The listing builds one solid part. Answer for the finished solid, in the listing's coordinates (mm). A direction names the side the tool comes from. Coordinates: 2 decimals unless noted, no trailing zeros.
(1) Which of the six approach directions +Z, -Z, +X, -X, +Y, -Y give full straight-line access (tool end or side, diameter ignored) to faces 5 (the flat face through (2, -9, 0)), 6 (the flat face through (31.1, -43.4, -1.5)), 7 (the cylindrical face through (2.405, -17.973, -1.521)), 8 (the flat face through (-2, -6, -0.5))?
(2) Straight lines are drawn through the part: line 1 (X direction, y = -34, z = -3.5); line 2 (X direction, y = -4.25, z = 1.4); line 3 (Z direction, x = 11, y = -18). For each, find the intervals that lie inside material, in ascending order.
(3) Given P1, Ø1, axis at x = 13, y = -19, coming from the -Z side; P2, Ø1.5, axis at y = -49, z = -6, coming from the +X side (3 decimals); P3, Ø2, axis at x = 1.5, y = -4.5, coming from the -Z side, each flat-ended and moving along its own axis, determine where each tip first touches the part or whether it passes through.
(4) For a pull along Y with two mould halves and no side action, classify faces 1 (the flat face through (25.423, -22.066, 0.042)), 2 (the cylindrical face through (-4.155, 0.748, 1.479)), 3 (the cylindrical face through (34.8, -48.2, -4)), 4 (the flat face through (35, -48, -10)) as +Y half, -Y half, draft (parallel to the pull), parting line (faces both ways), or undercut.
Autodesk Inventor part; units mm, degrees
ref_plane "YZ Plane" through (0, 0, 0) normal (1, 0, 0) x (0, 1, 0)
ref_plane "XY Plane" through (0, 0, 0) normal (0, 0, 1) x (1, 0, 0)
sketch "Skizze1" plane through (0, 0, 0) normal (0, 0, 1) x (1, 0, 0)
  line L0 (23.3115, -64.9198) -> (53.8426, -40.6536)
  circle A0 centre (0, -4.25) radius 6.5
  line L1 (43.6656, -48.7423) -> (33.4885, -56.8311)
  line L2 (33.4885, -56.8311) -> (-5.0885, -8.2944)
  line L3 (-5.0885, -8.2944) -> (5.0885, -0.2056)
  line L4 (5.0885, -0.2056) -> (43.6656, -48.7423)
  point P0 (0, 0)
  dimension "d0" = 13
extrude "Extrusion1" add sketch "Skizze1" along normal blind 3
sketch "Skizze2" plane through (43.6656, -48.7423, 0) normal (0.6222102, -0.7828502, 0) x (0.7828502, 0.6222102, 0)
  circle A0 centre (-17.7583, -20) radius 1.5
  circle A1 centre (4.7583, -20) radius 1.5
  circle A2 centre (-6.5, -0.5) radius 1.5
  line L0 (-23, -30.5) -> (10, -30.5)
  line L1 (10, -30.5) -> (10, -26.4615)
  arc A3 (11.0169, -22.0678) -> (10, -26.4615) centre (20, -26.4615) ccw
  arc A4 (11.0169, -22.0678) -> (-24.0169, -22.0678) centre (-6.5, -13.5) ccw
  arc A5 (-23, -26.4615) -> (-24.0169, -22.0678) centre (-33, -26.4615) ccw
  line L2 (-23, -26.4615) -> (-23, -30.5)
  line L3 (12.6833, -10) -> (-25.6833, -10)
  line L4 (-104.8912, -12) -> (94.8547, -12)
  line L5 (-13, 3) -> (0, 3)
  line L6 (3.8923, 3) -> (-16.8923, 3)
  line L7 (-21.75, -5.4123) -> (-19, -3.8246)
  line L8 (-19, -3.8246) -> (-16.25, -5.4123)
  line L9 (-16.25, -5.4123) -> (-16.25, -8.5877)
  line L10 (-16.25, -8.5877) -> (-19, -10.1754)
  line L11 (-19, -10.1754) -> (-21.75, -8.5877)
  line L12 (-21.75, -8.5877) -> (-21.75, -5.4123)
  line L13 (3.25, -5.4123) -> (6, -3.8246)
  line L14 (6, -3.8246) -> (8.75, -5.4123)
  line L15 (8.75, -5.4123) -> (8.75, -8.5877)
  line L16 (8.75, -8.5877) -> (6, -10.1754)
  line L17 (6, -10.1754) -> (3.25, -8.5877)
  line L18 (3.25, -8.5877) -> (3.25, -5.4123)
  circle A6 centre (-6.5, -13.5) radius 5
  point P0 (-3.8556, 0)
  dimension "d3" = 2
extrude "Extrusion2" add sketch "Skizze2" against normal blind 12 contours A4 L6 L5 L3 L16 L15 L14 L13 L18 L17 A6 L10 L9 L8 L7 L12 L11 | L11 L12 L7 L8 L9 L10 L3 | A6 L3 | L3 L17 L18 L13 L14 L15 L16
sketch "Skizze3" plane through (0, 0, 3) normal (0, 0, 1) x (1, 0, 0)
  line L0 (36.199, -39.3481) -> (5.0885, -0.2056)
  arc A0 (5.0885, -0.2056) -> (-5.0885, -8.2944) centre (0, -4.25) ccw
  line L1 (-5.0885, -8.2944) -> (26.022, -47.4369)
  line L2 (22.9749, -49.8587) -> (26.022, -47.4369)
  line L3 (30.4414, -59.2529) -> (22.9749, -49.8587)
  line L4 (46.7127, -46.3205) -> (30.4414, -59.2529)
  line L5 (46.7127, -46.3205) -> (39.2461, -36.9263)
  line L6 (36.199, -39.3481) -> (39.2461, -36.9263)
  line L7 (22.9749, -49.8587) -> (-5.0885, -8.2944)
  line L8 (39.2461, -36.9263) -> (5.0885, -0.2056)
  point P0 (0, 0)
extrude "Extrusion3" add sketch "Skizze3" against normal up to surface (3 mm away) contours L0 L8 L6 | L1 L2 L7
sketch "Skizze4" plane through (23.5594, -64.7228, -10) normal (0.6222102, -0.7828502, 0) x (0.7828502, 0.6222102, 0)
  line L0 (29.5756, 13) -> (8.791, 13)
  arc A0 (8.791, 13) -> (0, 0) centre (19.1833, -3.5) ccw
  line L1 (0, 0) -> (38.3667, 0)
  arc A1 (38.3667, 0) -> (29.5756, 13) centre (19.1833, -3.5) ccw
  arc A2 (17.7691, 10) -> (20.5975, 10) centre (19.1833, 9.5) ccw
  line L2 (17.7691, 10) -> (20.5975, 10)
  circle A3 centre (19.1833, 9.5) radius 1.5
  circle A4 centre (19.1833, 9.5) radius 3.5
  point P0 (21.8277, 10)
  dimension "d8" = 7
extrude "Extrusion4" cut sketch "Skizze4" against normal blind 12 contours A4 | L2 A2 | A3 L2
sketch "Skizze6" plane through (23.5594, -64.7228, -10) normal (0.6222102, -0.7828502, 0) x (0.7828502, 0.6222102, 0)
  circle A0 centre (19.1833, 9.5) radius 3.5
  line L0 (29.5756, 13) -> (19.1833, 13) construction
  arc A1 (8.791, 13) -> (0, 0) centre (19.1833, -3.5) ccw construction
  line L1 (0, 0) -> (38.3667, 0) construction
  arc A2 (38.3667, 0) -> (29.5756, 13) centre (19.1833, -3.5) ccw construction
  line L2 (15.6833, 13) -> (22.6833, 13)
  line L3 (22.6833, 13) -> (22.6833, 9.5)
  line L4 (22.6833, 9.5) -> (15.6833, 9.5)
  line L5 (15.6833, 9.5) -> (15.6833, 13)
  circle A3 centre (19.1833, 9.5) radius 3.5
  line L6 (19.1833, 13) -> (8.791, 13)
  point P0 (21.8277, 10)
  point P1 (21.0706, 13)
  point P2 (17.4651, 13)
extrude "Extrusion6" cut sketch "Skizze6" against normal up to surface (12 mm away) contours L4 A0 | A0 L2 L3 | A0 L5 L2 picked at (20.0662, 10.487)
sketch "Skizze7" plane through (36.199, -39.3481, 0) normal (-0.6222102, 0.7828502, 0) x (0.7828502, 0.6222102, 0)
  line L0 (-16.8923, -3) -> (-16.8923, 0)
  line L1 (-16.8923, 0) -> (-10, 0)
  line L2 (3.8923, 0) -> (3.8923, -3)
  arc A0 (3.8923, -3) -> (12.6833, 10) centre (-6.5, 13.5) ccw
  line L3 (12.6833, 10) -> (-25.6833, 10)
  arc A1 (-25.6833, 10) -> (-16.8923, -3) centre (-6.5, 13.5) ccw
  circle A2 centre (-19, 7) radius 1.5
  circle A3 centre (6, 7) radius 1.5
  line L4 (-3, 0.5) -> (-3, 0)
  line L5 (3.8923, 0) -> (-3, 0)
  line L6 (-10, 0) -> (-10, 0.5)
  arc A4 (-3, 0.5) -> (-10, 0.5) centre (-6.5, 0.5) ccw
  point P0 (-3.8556, 0)
extrude "Extrusion7" cut sketch "Skizze7" against normal through all contours A2 | A3
sketch "Skizze8" plane through (0, 0, 0) normal (0, 0, -1) x (-1, 0, 0)
  line L0 (-22.9749, -49.8587) -> (-28.3705, -45.5702)
  line L1 (-22.9749, -49.8587) -> (5.0885, -8.2944)
  arc A0 (5.0885, -8.2944) -> (-5.0885, -0.2056) centre (0, -4.25) ccw
  line L2 (-5.0885, -0.2056) -> (-39.2461, -36.9263)
  circle A1 centre (0, -4.25) radius 3.5
  line L3 (-33.8505, -41.2148) -> (-28.3705, -45.5702)
  line L4 (-39.2461, -36.9263) -> (-33.8505, -41.2148)
  point P0 (0, 0)
  dimension "d17" = 7
extrude "Extrusion8" add sketch "Skizze8" along normal blind 0.5 contours A1
chamfer "Fase1" distance 0.5 angle 45 1 edges at (3.5, -4.25, 0)
sketch "Skizze9" plane through (0, 0, 3) normal (0, 0, 1) x (1, 0, 0)
  circle A0 centre (0, -4.25) radius 3.5
  point P0 (0, 0)
hole "Bohrung1" at (0, -4.25, 3) direction (0, 0, -1) diameter 4 end through all
sketch "Skizze10" plane through (0, 0, 3) normal (0, 0, 1) x (1, 0, 0)
  circle A0 centre (24.2662, -34.7812) radius 3.5
  point P0 (0, 0)
  dimension "d30" = 7
extrude "Extrusion9" cut sketch "Skizze10" against normal through all
sketch "Skizze11" plane through (0, 0, 0) normal (0, 0, -1) x (-1, 0, 0)
  circle A0 centre (-24.2662, -34.7812) radius 3.5
  line L0 (-22.9749, -49.8587) -> (-28.3705, -45.5702)
  line L1 (-22.9749, -49.8587) -> (5.0885, -8.2944)
  arc A1 (5.0885, -8.2944) -> (-5.0885, -0.2056) centre (0, -4.25) ccw
  line L2 (-5.0885, -0.2056) -> (-39.2461, -36.9263)
  circle A2 centre (0, -4.25) radius 4
  arc A3 (-12.4206, -8.0879) -> (-0.9354, -17.2163) centre (0, -4.25) ccw
  line L3 (-22.9749, -49.8587) -> (5.0885, -8.2944)
  line L4 (-33.8505, -41.2148) -> (-28.3705, -45.5702)
  line L5 (-39.2461, -36.9263) -> (-33.8505, -41.2148)
  point P0 (0, 0)
  dimension "d33" = 13
extrude "Extrusion10" add sketch "Skizze11" along normal blind 5 contours L0 L4 L5 L2 A3 L1
fillet "Rundung1" radius 2 2 edges at (0.9354, -17.2163, -2.5) (12.4206, -8.0879, -2.5)
fillet "Rundung2" radius 2 8 edges at (2.4138, -17.9483, -5) (8.0887, -14.4271, -5) (12.8, -9.6934, -5) (26.8705, -23.6221, -5) (12.8073, -34.7996, -5) (22.9749, -49.8587, -1) (39.2461, -36.9263, -1) (31.1105, -43.3925, -5)
fillet "Rundung2" radius 4 2 edges at (49.8614, -36.1536, -10) (19.8261, -60.0257, -10)
properties part number "Mount_B" material "ABS-Kunststoff"
Model answer:
1. face 5: -Z
1. face 6: +Z
1. face 7: -Z, -X
1. face 8: -Z, +X, -X, +Y
2. line 1: x = 12.34 to 20.85, 27.68 to 36.44, 42.93 to 45.03
2. line 2: x = -6.5 to -2, 2 to 8.85
2. line 3: z = -5 to 3
3. P1: stops at z = -5
3. P2: stops at x = 44.285
3. P3: stops at z = -0.5
4. face 1: +Y half
4. face 2: parting line
4. face 3: undercut
4. face 4: draft
